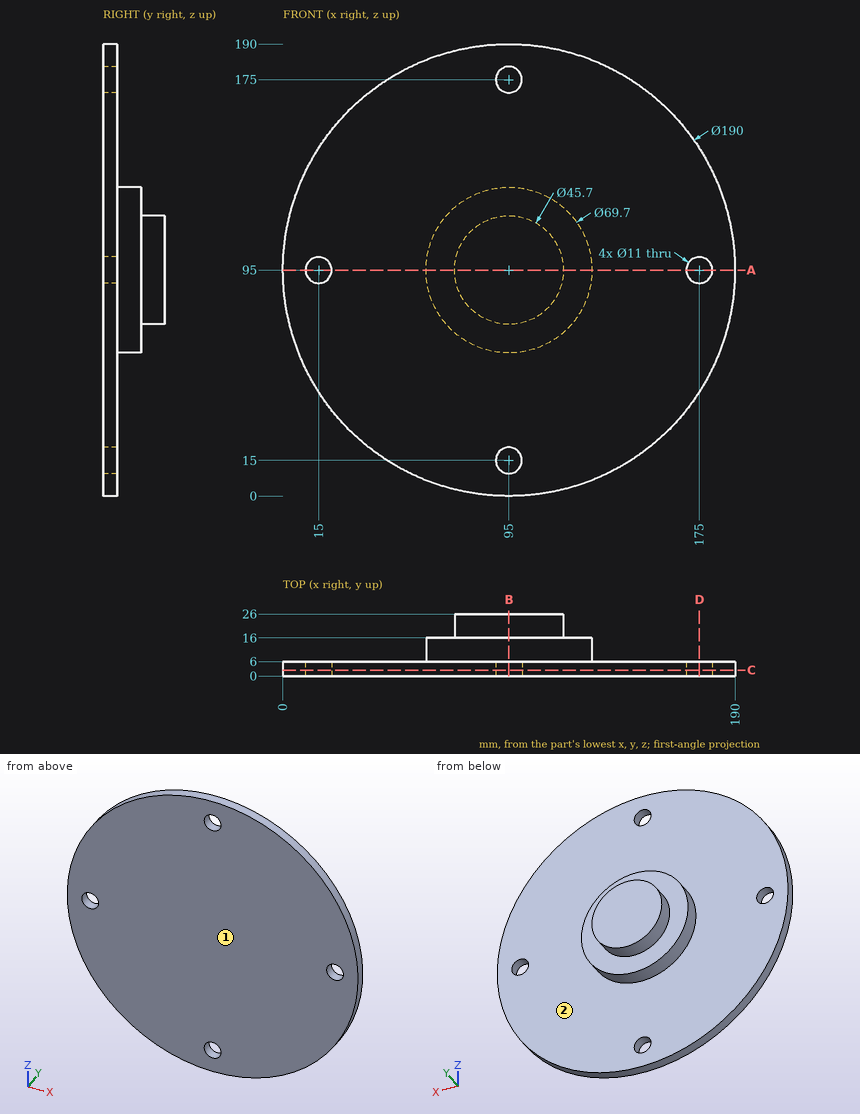
Part print with two shaded views. Sizes in mm from the minimum x, y, z corner. A direction names the side the tool comes from. Give positions to 0.01 mm unless a question says otherwise; leave off trailing zeros. Order: outer loops, then holes, each group sorted by start corner. A loop starts at its lowest first (then second) coordinate and runs counter-clockwise, first axis right, second up.
(1) Saw through at B-B, the plane x = 95. Give the cut face in (y, z), then the cut area to 3 significant figures.
(2) Tool access for the marked faces 1 and 2: list every direction of +Z, -Z, +X, -X, +Y, -Y with a clear straight run to the whole face (end or side of a thin tool).
(3) Saw through at C-C, the plane y = 2.5. Give the cut face in (x, z).
(4) Saw through at D-D, the plane x = 175. Give the cut face in (y, z).
(5) Drill centre lines: L1, parallel to Y at x = 85, z = 172; L2, parallel to X at y = 2.85, z = 175; L3, parallel to Y at x = 117, z = 70.5. Where is each one in solid material? Low to high.
(6) Flat gauge pins, fed straight in: pin 1 (3 mm diameter, centred on x = 102, z = 129, fed in from +Y); pin 2 (6.5 mm diameter, centred on x = 95, z = 15, fed in from -Y); pin 3 (17.5 mm diameter, centred on x = 15, z = 95, fed in from -Y); pin 4 (2 mm diameter, centred on y = 21, z = 90.5, fed in from -X). Where does each tip first touch, or does it go through?
(7) Saw through at A-A, the plane z = 95. Give the cut face in (x, y), then the cut area to 3 significant figures.
Results found:
1. outline: (0, 0) - (6, 0) - (6, 9.5) - (0, 9.5) - close; (0, 20.5) - (6, 20.5) - (6, 60.15) - (16, 60.15) - (16, 72.15) - (26, 72.15) - (26, 117.85) - (16, 117.85) - (16, 129.85) - (6, 129.85) - (6, 169.5) - (0, 169.5) - close; (0, 180.5) - (6, 180.5) - (6, 190) - (0, 190) - close
1. area: 2,160 mm2
2. face 1: +Z, -Z, +X, -X, -Y
2. face 2: +Y
3. outline: circle Ø190 at (95, 95); hole circle Ø11 at (15, 95); hole circle Ø11 at (95, 15); hole circle Ø11 at (95, 175); hole circle Ø11 at (175, 95)
4. outline: (0, 43.77) - (6, 43.77) - (6, 89.5) - (0, 89.5) - close; (0, 100.5) - (6, 100.5) - (6, 146.23) - (0, 146.23) - close
5. L1: y = 0 to 6
5. L2: x = 43.77 to 89.5, 100.5 to 146.23
5. L3: y = 0 to 16
6. pin 1: stops at y = 16
6. pin 2: passes through
6. pin 3: stops at y = 0
6. pin 4: stops at x = 72.42
7. outline: (0, 0) - (9.5, 0) - (9.5, 6) - (0, 6) - close; (20.5, 0) - (169.5, 0) - (169.5, 6) - (129.85, 6) - (129.85, 16) - (117.85, 16) - (117.85, 26) - (72.15, 26) - (72.15, 16) - (60.15, 16) - (60.15, 6) - (20.5, 6) - close; (180.5, 0) - (190, 0) - (190, 6) - (180.5, 6) - close
7. area: 2,160 mm2
